For this review, use the dimensioned drawing (mm, ordinates from the lowest corner) and the shaded views. A direction names the side the tool comes from. Coordinates: 2 decimals unless noted, no trailing zeros. Loops run counter-clockwise (first coordinate to the right, second up) from the corner with the lowest first, then second, coordinate; pieces in that order, holes last. Notation, with made-up numbers: (77.25, 11) - (95.25, 11) arc R35 ccw to (95.25, 48) - close; hole circle Ø9 at (38, 62). An arc over 180 degrees is marked (long way). Return JSON: item names as keys, results as strings. Group by question number.
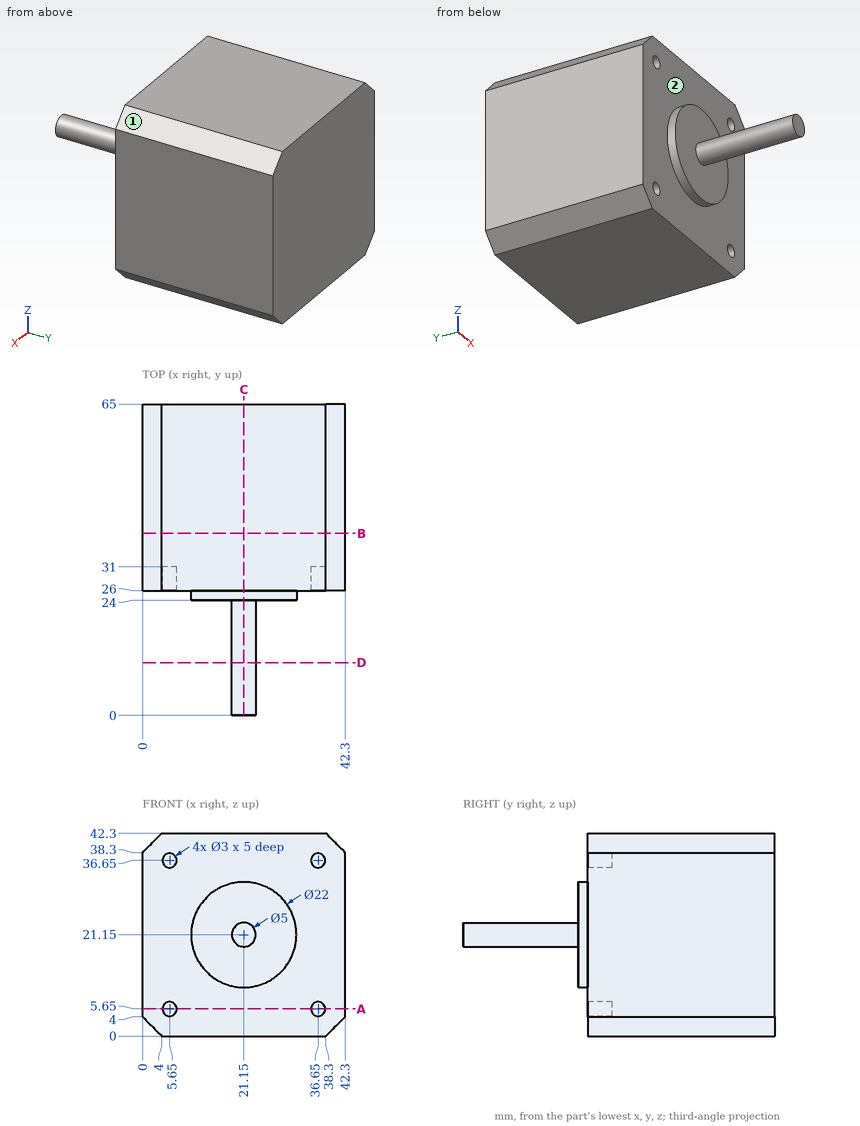
Item 1: Add section C-C (x = 21.15). State the section outline as (y, z) points, then the cut area to 3 significant figures.
Item 2: Add section A-A (z = 5.65). State the section outline as (x, y) points.
Item 3: To check wall thickness, follow line 1 (Z direction, x = 36.65, y = 29.2); line 2 (Y direction, x = 20.5, z = 36.5); line 3 (Z direction, x = 36, y = 29). State the ranges of each line that lie inside material, in increasing order. Write a range as from..to.
Item 4: Add section D-D (y = 11). State the section outline as (x, z) points, then the cut area to 3 significant figures.
Item 5: For the marked faces 1 and 2, list the 3-axis set-ups (+Z, -Z, +X, -X, +Y, -Y) from which the entire face can be reached by the end or side of a thin tool; tool diameter is ignored.
Item 6: Add section B-B (y = 38). State the section outline as (x, z) points, then the cut area to 3 significant figures.
Item 7: For P1, Ø0.9, axis at x = 37, z = 37, coming from the -Y side; P2, Ø2, axis at x = 22.5, y = 15, coming from the +Z side, all flat-tipped, find the tip position at first contact; note any pin that passes through.
Answers below:
{
 "1": {"outline": "(0, 18.65) - (24, 18.65) - (24, 10.15) - (26, 10.15) - (26, 0) - (65, 0) - (65, 42.3) - (26, 42.3) - (26, 32.15) - (24, 32.15) - (24, 23.65) - (0, 23.65) - close", "area": "1,810 mm^2"},
 "2": {"outline": "(0, 26) - (4.15, 26) - (4.15, 31) - (7.15, 31) - (7.15, 26) - (35.15, 26) - (35.15, 31) - (38.15, 31) - (38.15, 26) - (42.3, 26) - (42.3, 65) - (0, 65) - close"},
 "3": {"line 1": "z = 0..4.15, 7.15..35.15, 38.15..42.3", "line 2": "y = 26..65", "line 3": "z = 0..4.3, 7..35.3, 38..42.3"},
 "4": {"outline": "circle Ø5 at (21.15, 21.15)", "area": "19.6 mm^2"},
 "5": {"face 1": "+Z, +X, +Y, -Y", "face 2": "-Y"},
 "6": {"outline": "(0, 4) - (4, 0) - (38.3, 0) - (42.3, 4) - (42.3, 38.3) - (38.3, 42.3) - (4, 42.3) - (0, 38.3) - close", "area": "1,760 mm^2"},
 "7": {"P1": "stops at y = 31", "P2": "stops at z = 23.63"}
}
